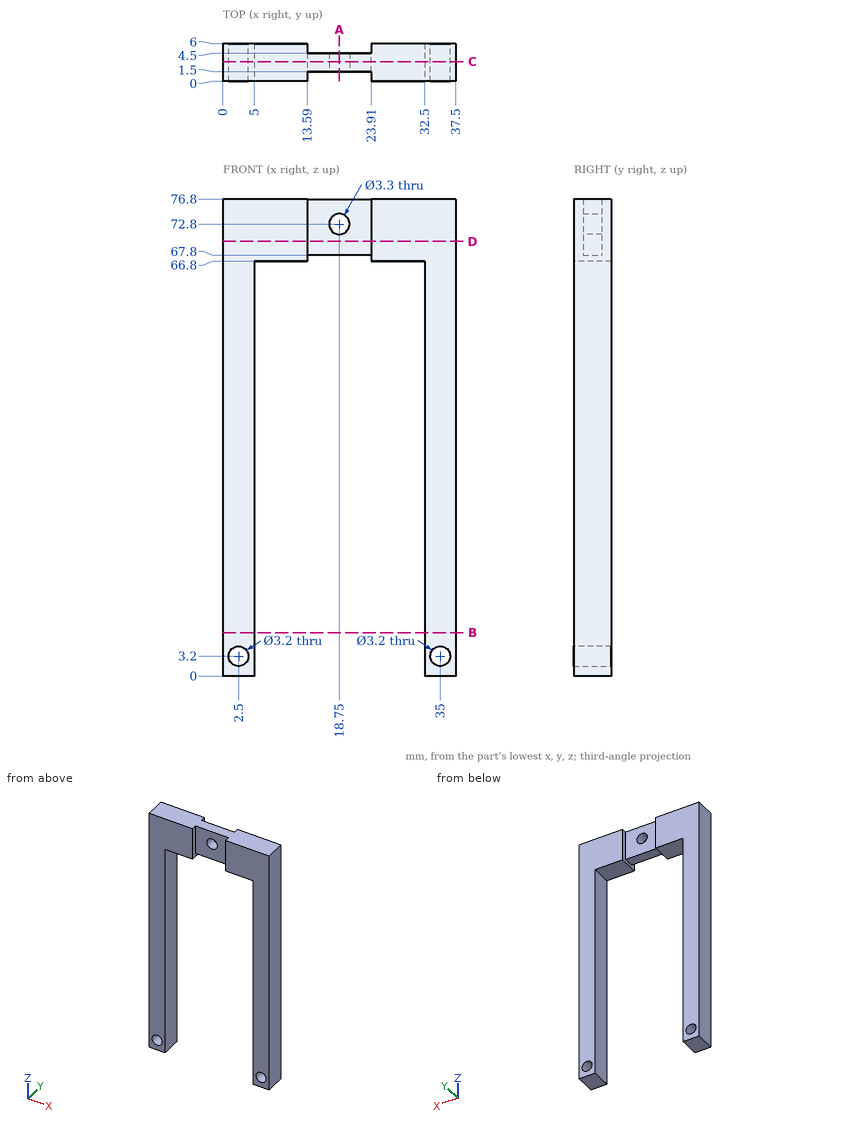
Answer from the drawing. Dimensions are ordinates in mm from the lowest x, y and z of the part. Give positions to 0.01 mm unless a question says otherwise; leave off trailing zeros. Order: outer loops, then holes, each group sorted by start corner. A loop starts at its lowest first (then second) coordinate and runs counter-clockwise, first axis right, second up.
(1) Find section D-D (z = 70). Give the vertices of the cut face in (x, y).
(2) Find section A-A (x = 18.75). Give the vertices of the cut face in (y, z).
(3) Given pin 1 (3 mm diameter, centred on x = 18.75, z = 72.8, fed in from +Y); pin 2 (2.5 mm diameter, centred on x = 21, z = 73, fed in from +Y); pin 3 (1.8 mm diameter, centred on x = 29, y = 4, fed in from -Z); pin 4 (1.5 mm diameter, centred on x = 21, y = 3, fed in from -Z), each flat-ended and moving along its own axis, determine where each tip first touches the part or whether it passes through.
(4) Find section C-C (y = 3.15). Give the vertices of the cut face in (x, z).
(5) Straight lines are drawn through the part: L1, parallel to X at y = 3.3, z = 72.8; L2, parallel to Z at x = 18.75, y = 2.3; L3, parallel to X at y = 0.85, z = 63. For each, find the intervals that lie inside material, in ascending order.
(6) Find section B-B (z = 7). Give the vertices of the cut face in (x, y).
Result sheet:
1. outline: (0, 0) - (13.59, 0) - (13.59, 1.5) - (23.91, 1.5) - (23.91, 0) - (37.5, 0) - (37.5, 6) - (23.91, 6) - (23.91, 4.5) - (13.59, 4.5) - (13.59, 6) - (0, 6) - close
2. outline: (1.5, 67.8) - (4.5, 67.8) - (4.5, 71.15) - (1.5, 71.15) - close; (1.5, 74.45) - (4.5, 74.45) - (4.5, 76.8) - (1.5, 76.8) - close
3. pin 1: passes through
3. pin 2: stops at y = 4.5
3. pin 3: stops at z = 66.8
3. pin 4: stops at z = 67.8
4. outline: (0, 0) - (5, 0) - (5, 66.8) - (13.59, 66.8) - (13.59, 67.8) - (23.91, 67.8) - (23.91, 66.8) - (32.5, 66.8) - (32.5, 0) - (37.5, 0) - (37.5, 76.8) - (0, 76.8) - close; hole circle Ø3.2 at (2.5, 3.2); hole circle Ø3.3 at (18.75, 72.8); hole circle Ø3.2 at (35, 3.2)
5. L1: x = 0 to 17.1, 20.4 to 37.5
5. L2: z = 67.8 to 71.15, 74.45 to 76.8
5. L3: x = 0 to 5, 32.5 to 37.5
6. outline: (0, 0) - (5, 0) - (5, 6) - (0, 6) - close; (32.5, 0) - (37.5, 0) - (37.5, 6) - (32.5, 6) - close
